Design review of the part built by this model. Coordinates are the model's own, in mm. Face numbers are marked on the shaded views. A direction names the side the tool comes from. Coordinates: 2 decimals unless noted, no trailing zeros. Write each loop counter-clockwise with the first axis right and the second up, starting at its lowest first coordinate (ties: lowest second). Pieces come first, ordered by that corner, then holes.
Q1. Add section A-A, the plane z = 33. Give the boundary of the cut face in (x, y), plus the area to 3 significant figures.
Q2. Add section B-B, the plane y = -4.25. Give the boundary of the cut face in (x, z), plus the area to 3 significant figures.
Q3. The part is to be moulded in two halves that separate along X. For the marked faces 3, 4, 5 and 6, say which applies: +X half, -X half, draft (parallel to the pull), parting line (faces both ways), or undercut.
Q4. Machinability: for the marked faces 1 and 2, which of the approach directions +Z, -Z, +X, -X, +Y, -Y give a long, thin tool a straight path to every point of the face, cutting with its end or side? Answer none if there is none.
Q5. Add section D-D, the plane z = 26.5. Give the boundary of the cut face in (x, y).
Q6. Clearance check with flat-ended pins moving along their axes: pin 1 Ø5 at (y, z) = (10, 45) entering from +X; pin 2 Ø2 at (x, y) = (49, 12.5) entering from +Z; pin 3 Ø8 at (x, z) = (50, 17.5) entering from -Y; pin 4 Ø1 at (x, y) = (-30.5, 1) entering from +Z. State where each tip first meets the part, or that it passes through.
Q7. To check wall thickness, follow probe 1 along Z at (x, y) = (2.11, 13.7); probe 2 along X at (y, z) = (0.5, 35.5); probe 3 along Y at (x, z) = (2.5, 13). State the ranges of each line that lie inside material, in increasing order.
Q8. Add section C-C, the plane x = -4.5. Give the boundary of the cut face in (y, z), plus the area to 3 significant figures.
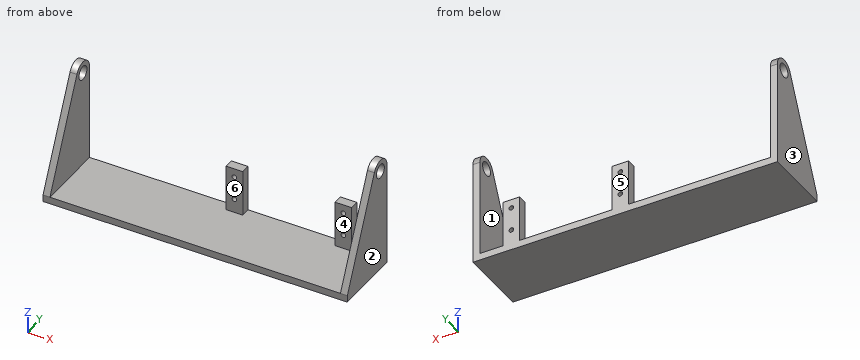
from build123d import *

# Parameters (mm, degrees)
F0_W     = 126
F0_H     = 30
F1_DEPTH = 3
F2_R     = 3
F2_W     = 30
F2_H     = 3
F3_DEPTH = 3
F4_W     = 7.26
F4_H     = 4
F5_DEPTH = 20
F6_R     = 1
F7_DEPTH = 4


# Not quite as in the source:
# - a pattern or mirror of a feature is missing from the dataset's text; its kind, count and spacing are read off the source's solid


with BuildPart() as f1:
    # F0 (on Top) → F1 (new body)
    with BuildSketch(Plane.XY):
        Rectangle(F0_W, F0_H)
    extrude(amount=F1_DEPTH)

    # F2 (on face) → F3 (join)
    with BuildSketch(Plane.YZ.offset(63)):
        with BuildLine():
            Line((-15, 3), (15, 3))
            Line((15, 3), (15, 45))
            ThreePointArc((15, 45), (11.0775660253, 49.8825046299), (5.4644594156, 47.1044884431))
            Line((5.4644594156, 47.1044884431), (-15, 3))
        make_face()
        with Locations((10, 45)):
            Circle(F2_R, mode=Mode.SUBTRACT)
        with Locations((0, 1.5)):
            Rectangle(F2_W, F2_H)
    f3 = extrude(amount=F3_DEPTH)

    # F3_copies: F3 across plane
    add(f3.mirror(Plane(origin=(0, 0, 0), x_dir=(0, 0, -1), z_dir=(-1, 0, 0))))

    # F4 (on face) → F5 (join)
    with BuildSketch(Plane.XY.offset(3)):
        with Locations((2.11, 13)):
            Rectangle(F4_W, F4_H)
        with Locations((49.37, 13)):
            Rectangle(F4_W, F4_H)
    extrude(amount=F5_DEPTH)

    # F6 (on face) → F7 (cut, through all)
    with BuildSketch(Plane(origin=(0, 15, 0), x_dir=(-1, 0, 0), z_dir=(0, 1, 0))):
        with Locations((-49.37, 19.17)):
            Circle(F6_R)
        with Locations((-49.37, 9)):
            Circle(F6_R)
        with Locations((-2.11, 19.17)):
            Circle(F6_R)
        with Locations((-2.11, 9)):
            Circle(F6_R)
    extrude(amount=-F7_DEPTH, mode=Mode.SUBTRACT)


solid = f1.part
Here are the results:
1. outline: (-66, -1.08) - (-63, -1.08) - (-63, 15) - (-66, 15) - close; (63, -1.08) - (66, -1.08) - (66, 15) - (63, 15) - close
1. area: 96.5 mm2
2. outline: (-66, 0) - (66, 0) - (66, 26.17) - (63, 26.17) - (63, 3) - (-63, 3) - (-63, 26.17) - (-66, 26.17) - close
2. area: 535 mm2
3. face 3: -X half
3. face 4: undercut
3. face 5: draft
3. face 6: undercut
4. face 1: +Z, +Y, -Y
4. face 2: +Z, -Z, +X, +Y, -Y
5. outline: (-66, -4.1) - (-63, -4.1) - (-63, 15) - (-66, 15) - close; (63, -4.1) - (66, -4.1) - (66, 15) - (63, 15) - close
6. pin 1: passes through
6. pin 2: stops at z = 23
6. pin 3: stops at y = 11
6. pin 4: stops at z = 3
7. probe 1: z = 0 to 8, 10 to 18.17, 20.17 to 23
7. probe 2: x = -66 to -63, 63 to 66
7. probe 3: y = 11 to 15
8. outline: (-15, 0) - (15, 0) - (15, 3) - (-15, 3) - close
8. area: 90.0 mm2
